Can you work these out from the model? Positions are in its coordinate system, mm. Give positions to 0.01 mm unless a question says otherwise; leave off trailing zeros. Order: outer loops, then holes, each group sorted by start corner. A loop starts at its lowest first (then second) coordinate and runs counter-clockwise, first axis right, second up. Notation, with made-up numbers: (67.5, 70.25) - (97.5, 70.25) arc R19 cw to (97.5, 82.25) - close; hole circle Ø7 at (34.5, 53). An arc over 180 degrees is marked (long way). Use one line per item in the form item = value. Start each with the question number.
1) Suppose I cut it at B-B, the plane z = 3.5. State how many separate pieces and enclosed holes the cut face has, and give its area (3 significant figures).
2) Please list where these lines run through material, in increasing order: probe 1 along X at (y, z) = (931.5, 6.75); probe 2 along X at (y, z) = (1080, 3.75); probe 3 along Y at (x, z) = (-524.5, 4.5).
3) Suppose I cut it at A-A, the plane y = 1066. Write out the boundary of the cut face in (x, z).
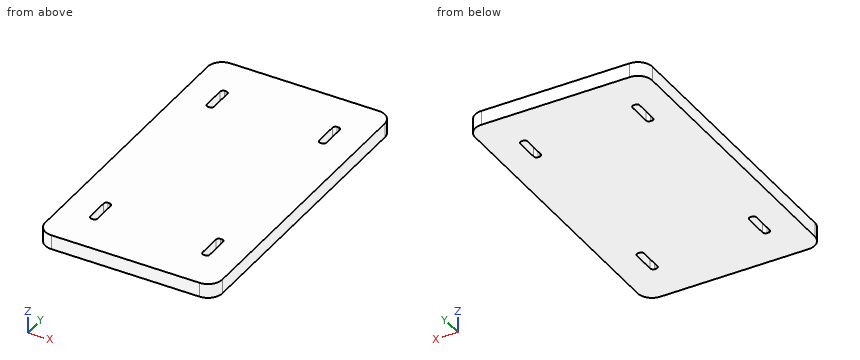
```python
from build123d import *

# Parameters (mm, degrees)
SALIENTE_EXTRUIR1_DEPTH = 10


with BuildPart() as part:
    # Croquis2 → Saliente-Extruir1 (new body)
    with BuildSketch(Plane.XY):
        with BuildLine():
            Line((-628.214587467, 894.02140807), (-525.214587467, 894.02140807))
            ThreePointArc((-525.214587467, 894.02140807), (-518.143519656, 896.950340259), (-515.214587467, 904.02140807))
            Line((-515.214587467, 904.02140807), (-515.214587467, 1099.02140807))
            ThreePointArc((-515.214587467, 1099.02140807), (-518.143519656, 1106.092475882), (-525.214587467, 1109.02140807))
            Line((-525.214587467, 1109.02140807), (-628.214587467, 1109.02140807))
            ThreePointArc((-628.214587467, 1109.02140807), (-635.285655279, 1106.092475882), (-638.214587467, 1099.02140807))
            Line((-638.214587467, 1099.02140807), (-638.214587467, 904.02140807))
            ThreePointArc((-638.214587467, 904.02140807), (-635.285655279, 896.950340259), (-628.214587467, 894.02140807))
        make_face()
        with BuildLine():
            Line((-537.214587467, 1081.52140807), (-538.214587467, 1081.52140807))
            ThreePointArc((-538.214587467, 1081.52140807), (-539.62880103, 1080.935621633), (-540.214587467, 1079.52140807))
            Line((-540.214587467, 1079.52140807), (-540.214587467, 1063.52140807))
            ThreePointArc((-540.214587467, 1063.52140807), (-539.62880103, 1062.107194508), (-538.214587467, 1061.52140807))
            Line((-538.214587467, 1061.52140807), (-537.214587467, 1061.52140807))
            ThreePointArc((-537.214587467, 1061.52140807), (-535.800373905, 1062.107194508), (-535.214587467, 1063.52140807))
            Line((-535.214587467, 1063.52140807), (-535.214587467, 1079.52140807))
            ThreePointArc((-535.214587467, 1079.52140807), (-535.800373905, 1080.935621633), (-537.214587467, 1081.52140807))
        make_face(mode=Mode.SUBTRACT)
        with BuildLine():
            Line((-616.214587467, 1061.52140807), (-615.214587467, 1061.52140807))
            ThreePointArc((-615.214587467, 1061.52140807), (-613.800373905, 1062.107194508), (-613.214587467, 1063.52140807))
            Line((-613.214587467, 1063.52140807), (-613.214587467, 1079.52140807))
            ThreePointArc((-613.214587467, 1079.52140807), (-613.800373905, 1080.935621633), (-615.214587467, 1081.52140807))
            Line((-615.214587467, 1081.52140807), (-616.214587467, 1081.52140807))
            ThreePointArc((-616.214587467, 1081.52140807), (-617.62880103, 1080.935621633), (-618.214587467, 1079.52140807))
            Line((-618.214587467, 1079.52140807), (-618.214587467, 1063.52140807))
            ThreePointArc((-618.214587467, 1063.52140807), (-617.62880103, 1062.107194508), (-616.214587467, 1061.52140807))
        make_face(mode=Mode.SUBTRACT)
        with BuildLine():
            Line((-535.214587467, 939.52140807), (-535.214587467, 923.52140807))
            ThreePointArc((-535.214587467, 923.52140807), (-535.800373905, 922.107194508), (-537.214587467, 921.52140807))
            Line((-537.214587467, 921.52140807), (-538.214587467, 921.52140807))
            ThreePointArc((-538.214587467, 921.52140807), (-539.62880103, 922.107194508), (-540.214587467, 923.52140807))
            Line((-540.214587467, 923.52140807), (-540.214587467, 939.52140807))
            ThreePointArc((-540.214587467, 939.52140807), (-539.62880103, 940.935621633), (-538.214587467, 941.52140807))
            Line((-538.214587467, 941.52140807), (-537.214587467, 941.52140807))
            ThreePointArc((-537.214587467, 941.52140807), (-535.800373905, 940.935621633), (-535.214587467, 939.52140807))
        make_face(mode=Mode.SUBTRACT)
        with BuildLine():
            Line((-616.214587467, 921.52140807), (-615.214587467, 921.52140807))
            ThreePointArc((-615.214587467, 921.52140807), (-613.800373905, 922.107194508), (-613.214587467, 923.52140807))
            Line((-613.214587467, 923.52140807), (-613.214587467, 939.52140807))
            ThreePointArc((-613.214587467, 939.52140807), (-613.800373905, 940.935621633), (-615.214587467, 941.52140807))
            Line((-615.214587467, 941.52140807), (-616.214587467, 941.52140807))
            ThreePointArc((-616.214587467, 941.52140807), (-617.62880103, 940.935621633), (-618.214587467, 939.52140807))
            Line((-618.214587467, 939.52140807), (-618.214587467, 923.52140807))
            ThreePointArc((-618.214587467, 923.52140807), (-617.62880103, 922.107194508), (-616.214587467, 921.52140807))
        make_face(mode=Mode.SUBTRACT)
    extrude(amount=SALIENTE_EXTRUIR1_DEPTH)


solid = part.part
```
Result sheet:
q1.separate_pieces = 1
q1.enclosed_holes = 4
q1.area = 26,000 mm²
q2.probe_1 = -638.21 to -618.21, -613.21 to -540.21, -535.21 to -515.21
q2.probe_2 = -638.21 to -618.16, -613.27 to -540.16, -535.27 to -515.21
q2.probe_3 = 894.05 to 1109
q3.outline = (-638.21, 0) - (-618.21, 0) - (-618.21, 10) - (-638.21, 10) - close; (-613.21, 0) - (-540.21, 0) - (-540.21, 10) - (-613.21, 10) - close; (-535.21, 0) - (-515.21, 0) - (-515.21, 10) - (-535.21, 10) - close
